```python
from build123d import *

# Parameters (mm, degrees)
SKETCH_R  = 1.5
PAD_DEPTH = 5
FILLET_R  = 3


with BuildPart() as part:
    # Sketch → Pad (new body)
    with BuildSketch(Plane.XY):
        Polygon((0, 45), (44.209009, 45), (55.310102, 75.5), (74.689898, 75.5), (85.790991, 45), (179.209009, 45), (190.310102, 75.5), (209.689898, 75.5), (220.790991, 45), (240.5, 45), (277.5, 8), (377.5, 8), (414.5, 45), (434.209009, 45), (445.310102, 75.5), (464.689898, 75.5), (475.790991, 45), (520, 45), (520, 37), (417.813708, 37), (380.813708, 0), (274.186292, 0), (237.186292, 37), (141.5, 37), (135.472158, 17), (129.527842, 17), (123.5, 37), (0, 37), align=None)
        with Locations((60, 70)):
            Circle(SKETCH_R, mode=Mode.SUBTRACT)
        with Locations((65, 70)):
            Circle(SKETCH_R, mode=Mode.SUBTRACT)
        with Locations((70, 70)):
            Circle(SKETCH_R, mode=Mode.SUBTRACT)
        with Locations((60, 65)):
            Circle(SKETCH_R, mode=Mode.SUBTRACT)
        with Locations((65, 65)):
            Circle(SKETCH_R, mode=Mode.SUBTRACT)
        with Locations((70, 65)):
            Circle(SKETCH_R, mode=Mode.SUBTRACT)
        with Locations((195, 70)):
            Circle(SKETCH_R, mode=Mode.SUBTRACT)
        with Locations((200, 70)):
            Circle(SKETCH_R, mode=Mode.SUBTRACT)
        with Locations((205, 70)):
            Circle(SKETCH_R, mode=Mode.SUBTRACT)
        with Locations((195, 65)):
            Circle(SKETCH_R, mode=Mode.SUBTRACT)
        with Locations((200, 65)):
            Circle(SKETCH_R, mode=Mode.SUBTRACT)
        with Locations((205, 65)):
            Circle(SKETCH_R, mode=Mode.SUBTRACT)
        with Locations((450, 70)):
            Circle(SKETCH_R, mode=Mode.SUBTRACT)
        with Locations((455, 70)):
            Circle(SKETCH_R, mode=Mode.SUBTRACT)
        with Locations((460, 70)):
            Circle(SKETCH_R, mode=Mode.SUBTRACT)
        with Locations((450, 65)):
            Circle(SKETCH_R, mode=Mode.SUBTRACT)
        with Locations((455, 65)):
            Circle(SKETCH_R, mode=Mode.SUBTRACT)
        with Locations((460, 65)):
            Circle(SKETCH_R, mode=Mode.SUBTRACT)
        with Locations((132.5, 21)):
            Circle(SKETCH_R, mode=Mode.SUBTRACT)
        Polygon((52.722432, 45), (58, 59.5), (72, 59.5), (77.277568, 45), align=None, mode=Mode.SUBTRACT)
        Polygon((187.722432, 45), (193, 59.5), (207, 59.5), (212.277568, 45), align=None, mode=Mode.SUBTRACT)
        Polygon((442.722432, 45), (448, 59.5), (462, 59.5), (467.277568, 45), align=None, mode=Mode.SUBTRACT)
    extrude(amount=PAD_DEPTH)

    # Fillet
    fillet_edges = [part.edges().sort_by_distance(p)[0] for p in [
        (0, 45, 2.5),
        (55.310102, 75.5, 2.5),
        (74.689898, 75.5, 2.5),
        (190.310102, 75.5, 2.5),
        (209.689898, 75.5, 2.5),
        (240.5, 45, 2.5),
        (277.5, 8, 2.5),
        (377.5, 8, 2.5),
        (414.5, 45, 2.5),
        (445.310102, 75.5, 2.5),
        (464.689898, 75.5, 2.5),
        (520, 45, 2.5),
        (520, 37, 2.5),
        (417.813708, 37, 2.5),
        (380.813708, 0, 2.5),
        (274.186292, 0, 2.5),
        (237.186292, 37, 2.5),
        (135.472158, 17, 2.5),
        (129.527842, 17, 2.5),
        (0, 37, 2.5),
        (187.722432, 45, 2.5),
        (193, 59.5, 2.5),
        (207, 59.5, 2.5),
        (212.277568, 45, 2.5),
        (52.722432, 45, 2.5),
        (58, 59.5, 2.5),
        (72, 59.5, 2.5),
        (77.277568, 45, 2.5),
        (442.722432, 45, 2.5),
        (448, 59.5, 2.5),
        (462, 59.5, 2.5),
        (467.277568, 45, 2.5),
    ]]
    fillet(fillet_edges, radius=FILLET_R)


solid = part.part
```
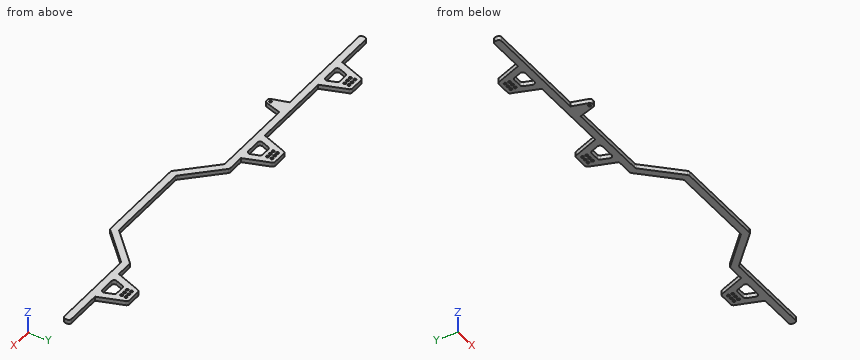
CAD build for the part. Positions are in the model's coordinates, mm. Coordinates: 2 decimals unless noted, no trailing zeros. Write each loop counter-clockwise with the first axis right and the second up, starting at its lowest first coordinate (ties: lowest second). Pieces come first, ordered by that corner, then holes.
(1) Cut at B-B, the plane x = 304. List the corners of the cut face in (y, z).
(2) Cut at C-C, the plane x = 471. List the corners of the cut face in (y, z).
(3) Flat gauge pins, fed straight in: pin 1 (2.5 mm diameter, centred on x = 205, y = 70, fed in from -Z); pin 2 (1 mm diameter, centred on x = 435, z = 4, fed in from -Y); pin 3 (1 mm diameter, centred on y = 21, z = 2.5, fed in from +X); pin 4 (3 mm diameter, centred on x = 133, z = 3.5, fed in from +Y). Where does each tip first touch, or does it go through?
(4) Cut at A-A, the plane z = 0.85. Count the separate pieces of the cut face and the enclosed holes in it, and give its area (3 significant figures).
(5) Drill centre lines: probe 1 along Y at (x, z) = (195, 1.25); probe 2 along Y at (x, z) = (63, 4.7); probe 3 along X at (y, z) = (49.5, 0.7). Where is each one in solid material? Low to high.
Geometry says:
1. outline: (0, 0) - (8, 0) - (8, 5) - (0, 5) - close
2. outline: (37, 0) - (58.16, 0) - (58.16, 5) - (37, 5) - close
3. pin 1: passes through
3. pin 2: stops at y = 37
3. pin 3: stops at x = 402.31
3. pin 4: stops at y = 45
4. separate pieces: 1
4. enclosed holes: 22
4. area: 6,480 mm2
5. probe 1: y = 37 to 45, 59.5 to 63.5, 66.5 to 68.5, 71.5 to 75.5
5. probe 2: y = 37 to 45, 59.5 to 75.5
5. probe 3: x = 45.85 to 54.36, 75.64 to 84.15, 180.85 to 189.36, 210.64 to 219.15, 435.85 to 444.36, 465.64 to 474.15
